CAD build for the part. Positions are in the model's coordinates, mm. A direction names the side the tool comes from. Coordinates: 2 decimals unless noted, no trailing zeros. Write each loop counter-clockwise with the first axis right and the second up, starting at its lowest first coordinate (ties: lowest second). Pieces come first, ordered by that corner, then holes. Notation, with made-up numbers: (1, 81) - (5, 81) arc R19 cw to (5, 92) - close; hole circle Ø7 at (-21.5, 31.25). An arc over 180 degrees is marked (long way). One line per question, with ' | ' between items. Start each with the question number.
1. Flat gauge pins, fed straight in: P1, Ø3, axis at x = -8, y = -22, coming from the +Z side; P2, Ø7.5, axis at x = -22, y = -10, coming from the +Z side; P3, Ø5, axis at y = -9.5, z = -8.5, coming from the -X side. Where does each tip first touch, or does it go through?
2. Probe line 1 (X direction, y = -23.75, z = -13); line 2 (X direction, y = -23.5, z = -6); line 3 (X direction, y = -23.5, z = -12). List the from-to ranges inside material, lowest first.
3. Band-saw the part on D-D, the plane x = 18. Write the cut outline in (y, z), then the cut area to 3 significant figures.
4. Two-plate mould, pull along Z, no slides. Class faces 3 (the flat face through (-1, -13, -40.056)), 4 (the flat face through (-1, 0, -9)), 5 (the flat face through (-27.816, -13, -2)): +Z half, -Z half, draft (parallel to the pull), parting line (faces both ways), or undercut.
5. Band-saw the part on A-A, the plane x = -22. Write the cut outline in (y, z).
6. Band-saw the part on B-B, the plane y = -20.5. Write the cut outline in (x, z), then the cut area to 3 significant figures.
7. Band-saw the part on C-C, the plane z = 14. Write the cut outline in (x, y).
8. Which spindle directions (+Z, -Z, +X, -X, +Y, -Y) get a long thin tool onto all of the face, cutting with end or side? Do faces 1 (the flat face through (-23, -13, -18.479)), 2 (the flat face through (-1, -25.4, -9)). Say none if no direction does.
from build123d import *

# Parameters (mm, degrees)
F0_R     = 5.310328
F0_W     = 9.508142
F0_H     = 34.190733
F0_W_2   = 21.241593
F0_H_2   = 10.317345
F1_DEPTH = 25.4


with BuildPart() as f1:
    # F0 (on Front) → F1 (new body)
    with BuildSketch(Plane.XZ):
        Polygon((76.368585, -40.055577), (0, 69.996111), (-75.761683, -40.055577), align=None)
        with Locations((-22.961151, -24.750333)):
            Circle(F0_R, mode=Mode.SUBTRACT)
        with Locations((-23.062301, -1.383293)):
            Rectangle(F0_W, F0_H, mode=Mode.SUBTRACT)
        with Locations((-0.4046, -1.517257)):
            Rectangle(F0_W_2, F0_H_2, mode=Mode.SUBTRACT)
        Polygon((11.430002, -18.47866), (27.411768, 15.712073), (37.997249, 10.662371), (22.054509, -23.444871), align=None, mode=Mode.SUBTRACT)
    extrude(amount=F1_DEPTH)


solid = f1.part
Filled in:
1) P1: stops at z = 60.55 | P2: stops at z = 43.49 | P3: stops at x = -55.76
2) line 1: x = -57.14 to -27.82, -18.31 to 13.99, 26.94 to 57.59 | line 2: x = -52.32 to -27.82, -18.31 to -11.03, 10.22 to 17.26, 30.21 to 52.74 | line 3: x = -56.45 to -27.82, -18.31 to 14.46, 27.4 to 56.9
3) outline: (-25.4, -40.06) - (0, -40.06) - (0, -21.55) - (-25.4, -21.55) - close; (-25.4, -4.42) - (0, -4.42) - (0, 44.06) - (-25.4, 44.06) - close | area: 1,700 mm²
4) face 3: -Z half | face 4: draft | face 5: undercut
5) outline: (-25.4, -40.06) - (0, -40.06) - (0, -29.97) - (-25.4, -29.97) - close; (-25.4, -19.53) - (0, -19.53) - (0, -18.48) - (-25.4, -18.48) - close; (-25.4, 15.71) - (0, 15.71) - (0, 38.04) - (-25.4, 38.04) - close
6) outline: (-75.76, -40.06) - (76.37, -40.06) - (0, 70) - close; hole circle Ø10.62 at (-22.96, -24.75); hole (-27.82, -18.48) - (-18.31, -18.48) - (-18.31, 15.71) - (-27.82, 15.71) - close; hole (-11.03, -6.68) - (10.22, -6.68) - (10.22, 3.64) - (-11.03, 3.64) - close; hole (11.43, -18.48) - (22.05, -23.44) - (38, 10.66) - (27.41, 15.71) - close | area: 7,300 mm²
7) outline: (-38.55, -25.4) - (-27.82, -25.4) - (-27.82, 0) - (-38.55, 0) - close; (-18.31, -25.4) - (26.61, -25.4) - (26.61, 0) - (-18.31, 0) - close; (31, -25.4) - (38.86, -25.4) - (38.86, 0) - (31, 0) - close
8) face 1: +Y, -Y | face 2: +Z, -Z, +X, -X, -Y
